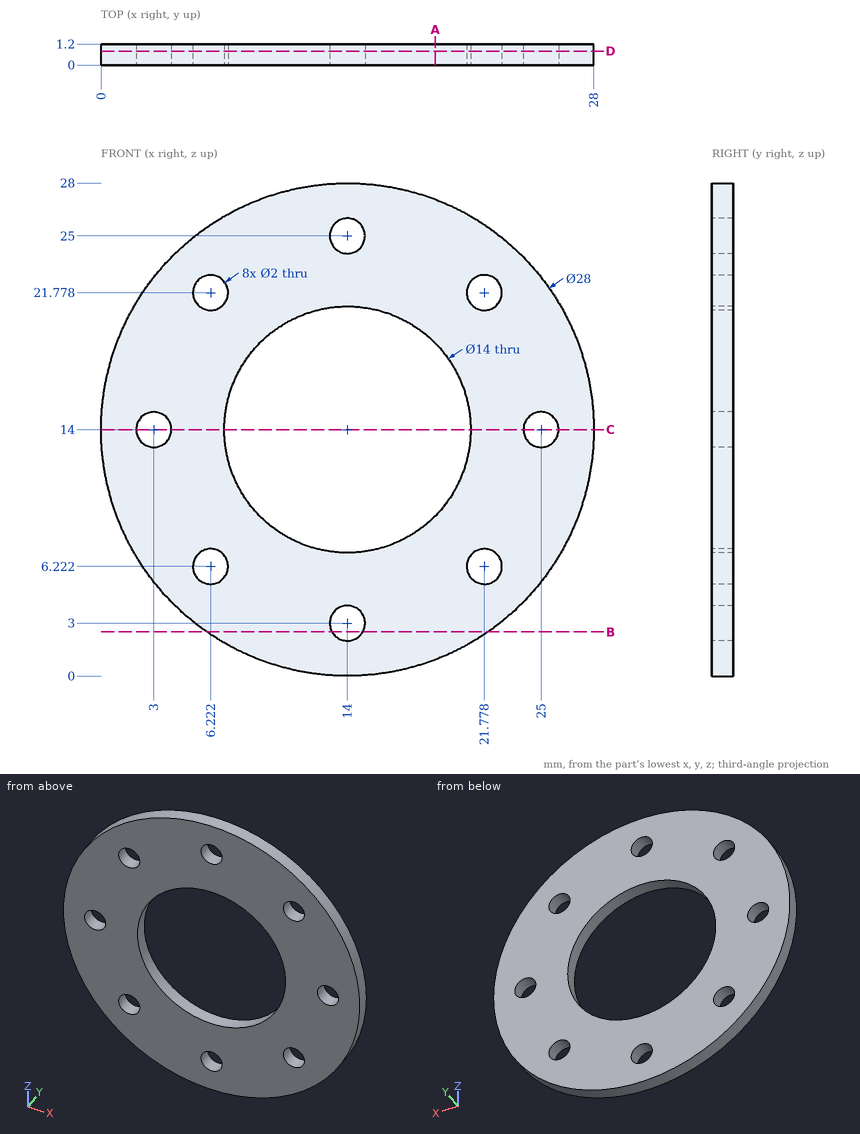
Answer from the drawing. Dimensions are ordinates in mm from the lowest x, y and z of the part. Give positions to 0.01 mm unless a question says otherwise; leave off trailing zeros. Order: outer loops, then holes, each group sorted by start corner. A loop starts at its lowest first (then second) coordinate and runs counter-clockwise, first axis right, second up.
Item 1: The part is cut by section D-D, the plane y = 0.8. Count the separate pieces of the cut face and the enclosed holes in it, and give its area (3 significant figures).
From the geometry:
separate pieces: 1
enclosed holes: 9
area: 437 mm2
Item 2: The part is cut by section C-C, the plane z = 14. Give the vertices of the cut face in (x, y), and give its area (3 significant figures).
From the geometry:
outline: (0, 0) - (2, 0) - (2, 1.2) - (0, 1.2) - close; (4, 0) - (7, 0) - (7, 1.2) - (4, 1.2) - close; (21, 0) - (24, 0) - (24, 1.2) - (21, 1.2) - close; (26, 0) - (28, 0) - (28, 1.2) - (26, 1.2) - close
area: 12.0 mm2
Item 3: Find the intervals of material crossed by probe 1 along Z at (x, y) = (14, 0.2); probe 2 along Z at (x, y) = (22, 0.1), in increasing order.
From the geometry:
probe 1: z = 0 to 2, 4 to 7, 21 to 24, 26 to 28
probe 2: z = 2.51 to 5.25, 7.2 to 20.8, 22.75 to 25.49
Item 4: The part is cut by section B-B, the plane z = 2.5. Give the vertices of the cut face in (x, y).
From the geometry:
outline: (6.02, 0) - (13.13, 0) - (13.13, 1.2) - (6.02, 1.2) - close; (14.87, 0) - (21.98, 0) - (21.98, 1.2) - (14.87, 1.2) - close
Item 5: The part is cut by section A-A, the plane x = 19. Give the vertices of the cut face in (y, z).
From the geometry:
outline: (0, 0.92) - (1.2, 0.92) - (1.2, 9.1) - (0, 9.1) - close; (0, 18.9) - (1.2, 18.9) - (1.2, 27.08) - (0, 27.08) - close
